```python
from build123d import *

# Parameters (mm, degrees)
SKETCH_1_R          = 10
EXTRUDE_1_DEPTH     = 40
SKETCH_3_R          = 2.5
CUT_EXTRUDE_8_DEPTH = 20
SKETCH_4_R          = 2.5
CUT_EXTRUDE_9_DEPTH = 20


with BuildPart() as part:
    # 草图1 → 凸台-拉伸1 (new body)
    with BuildSketch(Plane(origin=(0, 0, 0), x_dir=(1, 0, 0), z_dir=(0, 1, 0))):
        with Locations(Location((0, 0, 0), (0, 0, 270))):
            Circle(SKETCH_1_R)
    extrude(amount=EXTRUDE_1_DEPTH)

    # 草图3 → 切除-拉伸8 (cut)
    with BuildSketch(Plane(origin=(0, 40, 0), x_dir=(1, 0, 0), z_dir=(0, 1, 0))):
        with Locations(Location((0, 0, 0), (0, 0, 270))):
            Circle(SKETCH_3_R)
    extrude(amount=-CUT_EXTRUDE_8_DEPTH, mode=Mode.SUBTRACT)

    # 草图4 → 切除-拉伸9 (cut)
    with BuildSketch(Plane.XY):
        with Locations((0, 20)):
            Circle(SKETCH_4_R)
    extrude(amount=-CUT_EXTRUDE_9_DEPTH, mode=Mode.SUBTRACT)


solid = part.part
```
Input: part model. Units: mm. Frame: model coordinates. A direction names the side the tool comes from. Give positions to 0.01 mm unless a question says otherwise; leave off trailing zeros. Order: outer loops, then holes, each group sorted by start corner. A loop starts at its lowest first (then second) coordinate and runs counter-clockwise, first axis right, second up. Notation, with made-up numbers: (5.25, 34) -> (48.25, 34) arc R17 cw to (48.25, 52) -> close; hole circle Ø5 at (39.5, 60.25). An arc over 180 degrees is marked (long way). Write each question's results on one line, items separated by ' | '. Start each with the question number.
Item 1: Contact query for flat-ended pins moving along their axis: P1, Ø4, axis at x = 7.5, y = 14, coming from the -Z side; P2, Ø0.8, axis at x = 0, z = 1, coming from the +Y side. Output: stop coordinate, or through.
Item 2: Line query: line 1 (X direction, y = 27.75, z = 0); line 2 (Z direction, x = 1.25, y = 29); line 3 (Z direction, x = 2.25, y = 37). Output: solid intervals per line, ascending.
Item 3: Cut plane C-C on y = 8. Return the cut outline in (x, z), then the cut area to 3 significant figures.
Item 4: Cut plane B-B on z = -5. Return the cut outline in (x, y), then the cut area to 3 significant figures.
Item 5: Set-up query: faces 5 (the flat face through (0, 19, 0)), 6 (the flat face through (-2, 40, 2)). Return all of +Z, -Z, +X, -X, +Y, -Y with unobstructed straight access to the full face (end or side cutting, diameter ignored); none if empty.
Item 6: Mould query, pull axis Y, two halves, no side actions, for faces 1 (the cylindrical face through (-0.54, 17.56, -4.93)), 2 (the flat face through (0, 0, 0)), 3 (the cylindrical face through (0.751, 30.14, 2.385)), 4 (the flat face through (0, 20, 1)). Classes: pulls with the +Y half, pulls with the -Y half, needs draft (parallel to the pull), parting line crosses it, or undercut.
Item 7: Cut plane A-A on x = 0. Return the cut outline in (y, z).
Item 8: Cut plane D-D on z = 0.5. Return the cut outline in (x, y).
Established:
1) P1: z = -8.35 | P2: y = 20
2) line 1: -10 to -2.5, 2.5 to 10 | line 2: -9.92 to -2.17, 2.17 to 9.92 | line 3: -9.74 to -1.09, 1.09 to 9.74
3) outline: circle Ø20 at (0, 0) | area: 314 mm^2
4) outline: (-8.66, 0) -> (8.66, 0) -> (8.66, 40) -> (-8.66, 40) -> close; hole circle Ø5 at (0, 20) | area: 673 mm^2
5) face 5: -Z, +Y | face 6: +Z, -Z, +X, -X, +Y
6) face 1: undercut | face 2: pulls with the -Y half | face 3: needs draft | face 4: pulls with the +Y half
7) outline: (0, -10) -> (17.5, -10) -> (17.5, 0) -> (20, 0) -> (20, 2.5) -> (40, 2.5) -> (40, 10) -> (0, 10) -> close; (22.5, -10) -> (40, -10) -> (40, -2.5) -> (22.5, -2.5) -> close
8) outline: (-9.99, 0) -> (9.99, 0) -> (9.99, 40) -> (2.45, 40) -> (2.45, 20) -> (-2.45, 20) -> (-2.45, 40) -> (-9.99, 40) -> close
